from build123d import *

# Parameters (mm, degrees)
SKETCH1_R           = 4.25
SKETCH1_R_2         = 1.5
BOSS_EXTRUDE1_DEPTH = 12
FILLET1_R           = 2


with BuildPart() as part:
    # Sketch1 → Boss-Extrude1 (new body)
    with BuildSketch(Plane(origin=(0, 0, 0), x_dir=(1, 0, 0), z_dir=(0, 1, 0))):
        Polygon((0, 0), (170, 0), (170, 110), (125, 110), (125, 90), (45, 90), (45, 110), (0, 110), align=None)
        with Locations(Location((155, 10, 0), (0, 0, 270))):
            Circle(SKETCH1_R, mode=Mode.SUBTRACT)
        with Locations(Location((15, 10, 0), (0, 0, 90))):
            Circle(SKETCH1_R, mode=Mode.SUBTRACT)
        with Locations(Location((5, 104, 0), (0, 0, 270))):
            Circle(SKETCH1_R_2, mode=Mode.SUBTRACT)
        with Locations(Location((35, 104, 0), (0, 0, 270))):
            Circle(SKETCH1_R_2, mode=Mode.SUBTRACT)
        with Locations(Location((165, 104, 0), (0, 0, 90))):
            Circle(SKETCH1_R_2, mode=Mode.SUBTRACT)
        with Locations(Location((135, 104, 0), (0, 0, 90))):
            Circle(SKETCH1_R_2, mode=Mode.SUBTRACT)
    extrude(amount=BOSS_EXTRUDE1_DEPTH)

    # Fillet1
    fillet1_edges = [part.edges().sort_by_distance(p)[0] for p in [
        (45, 6, -90),
        (125, 6, -90),
        (170, 6, 0),
        (0, 6, 0),
    ]]
    fillet(fillet1_edges, radius=FILLET1_R)


solid = part.part
Design review of the part built by this model. Coordinates are the model's own, in mm. A direction names the side the tool comes from. Give positions to 0.01 mm unless a question says otherwise; leave off trailing zeros. Loops run counter-clockwise (first coordinate to the right, second up) from the corner with the lowest first, then second, coordinate; pieces in that order, holes last. Notation, with made-up numbers: (70.5, 68.5) - (107.5, 68.5) arc R22 ccw to (107.5, 78.5) - close; hole circle Ø7 at (25.25, 84.25). An arc over 180 degrees is marked (long way). Use CSV: the item, a comma, the result in double quotes. Start each with the question number.
1. Machinability: for faces 5 (the flat face through (125, 6, -101)), 6 (the flat face through (84, 6, 0)), which of the approach directions +Z, -Z, +X, -X, +Y, -Y give a long, thin tool a straight path to every point of the face, cutting with its end or side? Answer none if there is none.
2. Insertion check: P1, Ø1.5, axis at x = 86, y = 10.5, coming from the -Z side. The pin has a flat end and moves straight along its axis. Give the tip position at first contact, or say it passes through.
3. Add section D-D (y = 4.5). State the section outline as (x, z) points.
4. Add section B-B (z = -98.5). State the section outline as (x, y) points.
5. Add section C-C (z = -10). State the section outline as (x, y) points, plus the area to 3 significant figures.
6. Add section A-A (x = 15). State the section outline as (y, z) points.
7. Draft analysis for pull direction X (two halves, no side actions). For faces 1 (the cylindrical face through (17.59, 5.92, -6.63)), 2 (the flat face through (170, 6, -55)), 3 (the flat face through (148, 6, -110)), 4 (the cylindrical face through (159.214, 5.916, -10.553)), state which applies: released by +X, released by -X, zero draft, split by the parting line, or undercut.
8. Wall thickness on L1, parallel to X at y = 4.25, z = -10; L2, parallel to X at y = 4.5, z = -104; L3, parallel to X at y = 1.25, z = -97: over which ranges is each line inside the solid? List them lowest first.
Results found:
1,face 5,"-Z, +Y, -Y"
1,face 6,"+Z, +X, -X, +Y, -Y"
2,P1,"stops at z = -90"
3,outline,"(0, -110) - (45, -110) - (45, -92) arc R2 cw to (47, -90) - (123, -90) arc R2 cw to (125, -92) - (125, -110) - (170, -110) - (170, -2) arc R2 ccw to (168, 0) - (2, 0) arc R2 ccw to (0, -2) - close; hole circle Ø3 at (5, -104); hole circle Ø8.5 at (15, -10); hole circle Ø3 at (35, -104); hole circle Ø3 at (135, -104); hole circle Ø8.5 at (155, -10); hole circle Ø3 at (165, -104)"
4,outline,"(0, 0) - (45, 0) - (45, 12) - (0, 12) - close; (125, 0) - (170, 0) - (170, 12) - (125, 12) - close"
5,outline,"(0, 0) - (10.75, 0) - (10.75, 12) - (0, 12) - close; (19.25, 0) - (150.75, 0) - (150.75, 12) - (19.25, 12) - close; (159.25, 0) - (170, 0) - (170, 12) - (159.25, 12) - close"
5,area,"1,840 mm²"
6,outline,"(0, -110) - (12, -110) - (12, -14.25) - (0, -14.25) - close; (0, -5.75) - (12, -5.75) - (12, 0) - (0, 0) - close"
7,face 1,"undercut"
7,face 2,"released by +X"
7,face 3,"zero draft"
7,face 4,"undercut"
8,L1,"x = 0 to 10.75, 19.25 to 150.75, 159.25 to 170"
8,L2,"x = 0 to 3.5, 6.5 to 33.5, 36.5 to 45, 125 to 133.5, 136.5 to 163.5, 166.5 to 170"
8,L3,"x = 0 to 45, 125 to 170"
